```python
from build123d import *

# Parameters (mm, degrees)
BOSS_EXTRUDE1_DEPTH = 6
CUT_EXTRUDE2_DEPTH  = 3.5
SKETCH5_R           = 1.75
CUT_EXTRUDE3_DEPTH  = 4


with BuildPart() as part:
    # Sketch2 → Boss-Extrude1 (new body)
    with BuildSketch(Plane(origin=(0, 0, 0), x_dir=(1, 0, 0), z_dir=(0, 1, 0))):
        Polygon((-27.5, -6), (-27.5, 6), (-27.5, 19.170673077), (-39.134615385, 19.170673077), (-39.134615385, -19.170673077), (-27.5, -19.170673077), align=None)
        Polygon((0, -6), (0, 0), (0, 6), (-27.5, 6), (-27.5, -6), align=None)
        Polygon((0, 6), (0, 0), (0, -6), (27.5, -6), (27.5, 6), align=None)
        Polygon((27.5, 19.170673077), (27.5, 6), (27.5, -6), (27.5, -19.170673077), (39.134615385, -19.170673077), (39.134615385, 19.170673077), align=None)
    extrude(amount=BOSS_EXTRUDE1_DEPTH)

    # Sketch3 → Cut-Extrude2 (cut)
    with BuildSketch(Plane(origin=(0, 6, 0), x_dir=(1, 0, 0), z_dir=(0, 1, 0))):
        with BuildLine():
            Line((-29.544200918, 3), (-29.544200918, -3))
            ThreePointArc((-29.544200918, -3), (-33.044200918, -6.5), (-36.544200918, -3))
            Line((-36.544200918, -3), (-36.544200918, 3))
            ThreePointArc((-36.544200918, 3), (-33.044200918, 6.5), (-29.544200918, 3))
        make_face()
    extrude(amount=-CUT_EXTRUDE2_DEPTH, mode=Mode.SUBTRACT)

    # Sketch5 → Cut-Extrude3 (cut)
    with BuildSketch(Plane(origin=(0, 2.5, 0), x_dir=(1, 0, 0), z_dir=(0, 1, 0))):
        with Locations(Location((-33.044200918, 3, 0), (0, 0, 270))):
            Circle(SKETCH5_R)
        with Locations(Location((-33.044200918, -3, 0), (0, 0, 270))):
            Circle(SKETCH5_R)
    extrude(amount=-CUT_EXTRUDE3_DEPTH, mode=Mode.SUBTRACT)


solid = part.part
```
The model under review builds one solid part; all positions refer to its coordinate system, in mm. A direction names the side the tool comes from. Round coordinates to 2 decimals unless told otherwise and drop trailing zeros. Write each loop counter-clockwise with the first axis right and the second up, starting at its lowest first coordinate (ties: lowest second). Pieces come first, ordered by that corner, then holes. Notation, with made-up numbers: M 25,-3.5 L 71,-3.5 A32 ccw 71,25.5 Z; hole C 58,37 d7. An arc over 180 degrees is marked long. Use CSV: the item, a comma, the result in double quotes. Start each with the question number.
(1) The part is to be moulded in two halves that separate along Z. For faces 1 (the face through (-36.544, 4, 0)), 2 (the face through (-39.135, 3, 0)), 3 (the face through (-33, 3, -19.171)), 4 (the face through (-33, 3, 19.171)), say which applies: +Z half, -Z half, draft (parallel to the pull), parting line (faces both ways), or undercut.
(2) We need section C-C, the plane x = 21.5. State the section outline as (y, z) points.
(3) We need section A-A, the plane z = -15.5. State the section outline as (x, y) points.
(4) We need section B-B, the plane y = 3.2. State the section outline as (x, z) points.
(5) Clearance check with flat-ended pins moving along their axes: P1, Ø3.5, axis at x = -34.5, z = -1.5, coming from the +Y side; P2, Ø3, axis at x = -9, y = 3, coming from the +Z side. State where each tip first meets the part, or that it passes through.
(6) For line 1 along X through (y, z) = (1.7, -3); line 2 along X through (y, z) = (0.9, 7.5); line 3 along Z through (x, y) = (-3.5, 4.25), list the stretches that pass through material, from the lowest coordinate up.
(7) Tool access review of faces 5 (the face through (0, 3, -6)), 6 (the face through (-27.5, 3, 13)), 7 (the face through (-33, 2.5, 0)): name each direction out of +Z, -Z, +X, -X, +Y, -Y from which nothing blocks a thin tool from reaching the whole face with its end or side.
Findings:
1,face 1,"undercut"
1,face 2,"draft"
1,face 3,"-Z half"
1,face 4,"+Z half"
2,outline,"M 0,-6 L 6,-6 L 6,6 L 0,6 Z"
3,outline,"M -39.13,0 L -27.5,0 L -27.5,6 L -39.13,6 Z; M 27.5,0 L 39.13,0 L 39.13,6 L 27.5,6 Z"
4,outline,"M -39.13,-19.17 L -27.5,-19.17 L -27.5,-6 L 27.5,-6 L 27.5,-19.17 L 39.13,-19.17 L 39.13,19.17 L 27.5,19.17 L 27.5,6 L -27.5,6 L -27.5,19.17 L -39.13,19.17 Z; hole M -36.54,-3 A3.5 ccw -29.54,-3 L -29.54,3 A3.5 ccw -36.54,3 Z"
5,P1,"y = 2.5"
5,P2,"z = 6"
6,line 1,"-39.13 to -34.79, -31.29 to 39.13"
6,line 2,"-39.13 to -27.5, 27.5 to 39.13"
6,line 3,"-6 to 6"
7,face 5,"-Z, +Y, -Y"
7,face 6,"+Z, +Y, -Y"
7,face 7,"+Y"
